Model file for the job. Use its own axes, mm. Face numbers are marked on the shaded views. A direction names the side the tool comes from. Coordinates: 2 decimals unless noted, no trailing zeros. Loops run counter-clockwise (first coordinate to the right, second up) from the corner with the lowest first, then second, coordinate; pieces in that order, holes last.
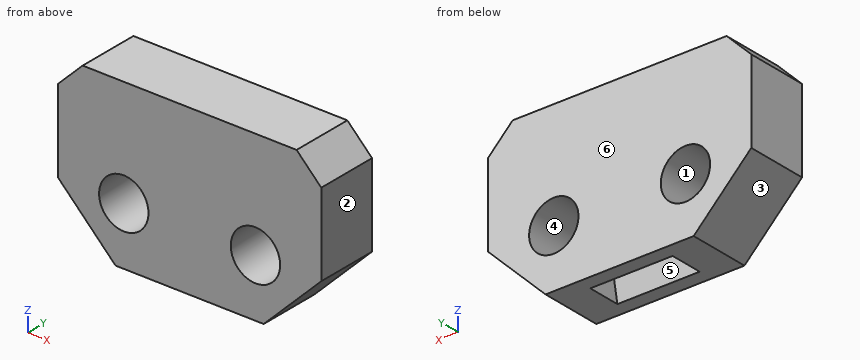
from build123d import *

# Parameters (mm, degrees)
F1_W     = 32
F1_H     = 20
F2_DEPTH = 7.5
F3_SIZE  = 7
F4_R     = 3
F5_DEPTH = 25
F6_SIZE  = 3
F7_W     = 10
F7_H     = 2
F8_DEPTH = 5
F9_SIZE2 = 0.99999
F9_SIZE  = 4.99999


# Not quite as in the source:
# - a fillet or chamfer is up to 0.001 mm smaller than in the source, because OpenCascade refuses the exact size


with BuildPart() as f2:
    # F1 (on Front) → F2 (new body)
    with BuildSketch(Plane.XZ):
        Rectangle(F1_W, F1_H)
    extrude(amount=F2_DEPTH)

    # F3
    f3_edges = [f2.edges().sort_by_distance(p)[0] for p in [
        (-16, -3.75, -10),
        (16, -3.75, -10),
    ]]
    chamfer(f3_edges, length=F3_SIZE)

    # F4 (on face) → F5 (cut)
    with BuildSketch(Plane.XZ.offset(7.5)):
        with Locations((-8, -3)):
            Circle(F4_R)
        with Locations((8, -3)):
            Circle(F4_R)
    extrude(amount=-F5_DEPTH, mode=Mode.SUBTRACT)

    # F6
    f6_edges = [f2.edges().sort_by_distance(p)[0] for p in [
        (16, -3.75, 10),
        (-16, -3.75, 10),
    ]]
    chamfer(f6_edges, length=F6_SIZE)

    # F7 (on face) → F8 (cut)
    with BuildSketch(Plane(origin=(0, 0, -10), x_dir=(1, 0, 0), z_dir=(0, 0, -1))):
        with Locations((0, 4.75)):
            Rectangle(F7_W, F7_H)
        with Locations((0, 2.75)):
            Rectangle(F7_W, F7_H)
    extrude(amount=-F8_DEPTH, mode=Mode.SUBTRACT)

    # F9 (size 5 and 1 in the source; OpenCascade refuses exactly that, so slightly less here)
    f9_edges = [f2.edges().sort_by_distance(p)[0] for p in [
        (0, -1.75, -5),
        (0, -5.75, -5),
    ]]
    chamfer(f9_edges, length=F9_SIZE, length2=F9_SIZE2)


solid = f2.part
Q1. Mould opens along Z. For the marked faces 1, 2, 3 and 4 say: +Z half, -Z half, draft (parallel to the pull), parting line (faces both ways), or undercut.
Answers:
face 1: undercut
face 2: draft
face 3: -Z half
face 4: undercut
Q2. Slice it at B-B (x = 8). List the corners of the cut face in (y, z).
Answers:
outline: (-7.5, -10) - (0, -10) - (0, -6) - (-7.5, -6) - close; (-7.5, 0) - (0, 0) - (0, 10) - (-7.5, 10) - close
Q3. Drill centre lines: line 1 (X direction, y = -1.5, z = -0.25); line 2 (Z direction, x = -8, y = -5.25); line 3 (X direction, y = -4, z = -1.5). Where is each one in solid material? Low to high.
Answers:
line 1: x = -16 to -9.2, -6.8 to 6.8, 9.2 to 16
line 2: z = -10 to -6, 0 to 10
line 3: x = -16 to -10.6, -5.4 to 5.4, 10.6 to 16
Q4. Slice it at A-A (y = -7). List the corners of the cut face in (x, z).
Answers:
outline: (-16, -3) - (-9, -10) - (9, -10) - (16, -3) - (16, 7) - (13, 10) - (-13, 10) - (-16, 7) - close; hole circle Ø6 at (-8, -3); hole circle Ø6 at (8, -3)
Q5. Slice it at D-D (y = -4). List the corners of the cut face in (x, z), and give its area (3 significant figures).
Answers:
outline: (-16, -3) - (-9, -10) - (-5, -10) - (-5, -5) - (5, -5) - (5, -10) - (9, -10) - (16, -3) - (16, 7) - (13, 10) - (-13, 10) - (-16, 7) - close; hole circle Ø6 at (-8, -3); hole circle Ø6 at (8, -3)
area: 475 mm2
Q6. Flat gauge pins, fed straight in: P1, Ø2, axis at x = 9, z = -8, coming from the +Y side; P2, Ø4.5, axis at y = -3, z = -8.5, coming from the +X side; P3, Ø3, axis at y = -3, z = -8.5, coming from the -X side. Where does each tip first touch, or does it go through?
Answers:
P1: stops at y = 0
P2: stops at x = 12.75
P3: stops at x = -12
Q7. Which spindle directions (+Z, -Z, +X, -X, +Y, -Y) get a long thin tool onto all of the face, cutting with end or side? Do the marked faces 5 and 6. Say none if no direction does.
Answers:
face 5: -Z
face 6: +Z, -Z, +X, -X, +Y
